```python
from build123d import *

# Parameters (mm, degrees)
F0_W      = 609.6
F0_H      = 609.6
F1_DEPTH  = 482.6
F2_T      = -12.7
F3_DEPTH  = 254
F4_T      = -12.7
F5_W      = 304.8
F5_H      = 609.6
F6_DEPTH  = 469.9
F7_T      = -12.7
F8_DEPTH  = 469.9
F9_DEPTH  = 342.9
F10_W     = 279.4
F10_H     = 457.2
F11_DEPTH = 596.9
F12_W     = 584.2
F12_H     = 330.2
F13_DEPTH = 596.9
F14_W     = 609.6
F14_H     = 1549.4
F15_DEPTH = 12.7


# Not quite as in the source:
# - a shell that OpenCascade refuses in one call is made with other operations: the cavity is built on its own and cut out


with BuildPart() as f1:
    # F0 (on Top) → F1 (new body)
    with BuildSketch(Plane.XY):
        with Locations((3.9980113506, 30.8666436833)):
            Rectangle(F0_W, F0_H)
    extrude(amount=F1_DEPTH)

    # F2
    f2_openings = [f1.faces().sort_by_distance(p)[0] for p in [
        (3.998011, -273.933356, 241.3),
    ]]
    offset(amount=F2_T, openings=f2_openings)

    # F3 (add): a face of the model
    f3_faces = [f1.faces().sort_by_distance(p)[0] for p in [
        (3.9980113506, 30.8666436833, 482.6),
    ]]
    extrude(f3_faces, amount=F3_DEPTH)

    # F4: a shell. OpenCascade refuses it in one call, so the cavity is built on its own and cut out:
    # the body offset inwards by the wall thickness, plus a prism from it out through each open face.
    f4_core = offset(f1.part, amount=F4_T, kind=Kind.INTERSECTION, mode=Mode.PRIVATE)
    f4_exits = [f4_core.faces().sort_by_distance(p)[0] for p in [
        (3.998011, -261.233356, 603.25),
    ]]
    add(f4_core, mode=Mode.SUBTRACT)
    extrude(f4_exits, amount=-F4_T, mode=Mode.SUBTRACT)

    # F5 (on face) → F6 (join)
    with BuildSketch(Plane.XY.offset(736.6)):
        with Locations((-148.4019886494, 30.8666436833)):
            Rectangle(F5_W, F5_H)
    extrude(amount=F6_DEPTH)

    # F7: a shell. OpenCascade refuses it in one call, so the cavity is built on its own and cut out:
    # the body offset inwards by the wall thickness, plus a prism from it out through each open face.
    f7_core = offset(f1.part, amount=F7_T, kind=Kind.INTERSECTION, mode=Mode.PRIVATE)
    f7_exits = [f7_core.faces().sort_by_distance(p)[0] for p in [
        (-148.401989, -261.233356, 965.2),
    ]]
    add(f7_core, mode=Mode.SUBTRACT)
    extrude(f7_exits, amount=-F7_T, mode=Mode.SUBTRACT)

    # F8 (add): a face of the model
    f8_faces = [f1.faces().sort_by_distance(p)[0] for p in [
        (156.3980113506, 30.8666436833, 736.6),
    ]]
    extrude(f8_faces, amount=F8_DEPTH)

    # F9 (add): a face of the model
    f9_faces = [f1.faces().sort_by_distance(p)[0] for p in [
        (3.9980113506, 30.8666436833, 1206.5),
    ]]
    extrude(f9_faces, amount=F9_DEPTH)

    # F10 (on face) → F11 (cut)
    with BuildSketch(Plane.XZ.offset(273.9333563167)):
        with Locations((156.3980113506, 965.2)):
            Rectangle(F10_W, F10_H)
    extrude(amount=-F11_DEPTH, mode=Mode.SUBTRACT)

    # F12 (on face) → F13 (cut)
    with BuildSketch(Plane.XZ.offset(273.9333563167)):
        with Locations((3.9980113506, 1371.6)):
            Rectangle(F12_W, F12_H)
    extrude(amount=-F13_DEPTH, mode=Mode.SUBTRACT)


with BuildPart() as f15:
    # F14 (on face) → F15 (new body)
    with BuildSketch(Plane.XZ.offset(273.9333563167)):
        with Locations((3.9980113506, 774.7)):
            Rectangle(F14_W, F14_H)
    extrude(amount=F15_DEPTH)


solid = f1.part
```
Geometry check sheet. Reference: the model listing, model coordinates, mm. A direction names the side the tool comes from. Coordinates: 2 decimals unless noted, no trailing zeros. Loops run counter-clockwise (first coordinate to the right, second up) from the corner with the lowest first, then second, coordinate; pieces in that order, holes last. Notation, with made-up numbers: (32, 9.25) - (79, 9.25) arc R12 cw to (79, 25.25) - close; hole circle Ø11 at (67, 60.25). An arc over 180 degrees is marked (long way). One line per item, written item: value. Start each with the question number.
(1) Material ranges on line 1 (Z direction, x = 16.5, y = 236); line 2 (Z direction, x = -234.5, y = 271); line 3 (X direction, y = 46, z = 982.5), recorded low to high. Write a range as [from, to].
(2) Cross-section at A-A on y = 174.5. Enter the section's corners in (x, z), plus the area to 3 significant figures.
(3) Depth check by flat-ended pin: P1, Ø12, axis at x = -165.5, z = 1171.5, coming from the -Y side. Enter the tip coordinate at first touch or a pass-through.
(4) Mould release check, pull along Z, two halves, no side actions. Record for faces 1 (the flat face through (0, 35, 0)), 2 (the flat face through (0, 322.967, 238)), 3 (the flat face through (0, 35, 1549.4)), 4 (the flat face through (-150, 29, 736.6)): released by +Z, released by -Z, zero draft, split by the parting line, or undercut.
(5) Tool access check on faces 5 (the flat face through (-300.802, 27, 764)), 6 (the flat face through (0, 20, 1536.7)). Record the directions out of +Z, -Z, +X, -X, +Y, -Y that give a thin tool (end or side, any length) a straight path to the whole face; none if there is none.
(6) Cross-section at B-B on x = 136.5. Enter the section's corners in (y, z), plus the area to 3 significant figures.
(7) Cross-section at C-C on z = 1247.5. Enter the section's corners in (x, y), plus the area to 3 significant figures.
Results below:
1. line 1: z = [0, 12.7], [469.9, 482.6], [723.9, 1206.5], [1536.7, 1549.4]
1. line 2: z = [0, 12.7], [469.9, 482.6], [723.9, 736.6], [1193.8, 1206.5], [1536.7, 1549.4]
1. line 3: x = [-300.8, -288.1], [-8.7, 16.7], [296.1, 308.8]
2. outline: (-300.8, 0) - (308.8, 0) - (308.8, 1549.4) - (-300.8, 1549.4) - close; hole (-288.1, 12.7) - (296.1, 12.7) - (296.1, 469.9) - (-288.1, 469.9) - close; hole (-288.1, 482.6) - (296.1, 482.6) - (296.1, 723.9) - (-288.1, 723.9) - close; hole (-288.1, 736.6) - (-8.7, 736.6) - (-8.7, 1193.8) - (-288.1, 1193.8) - close; hole (-288.1, 1206.5) - (296.1, 1206.5) - (296.1, 1536.7) - (-288.1, 1536.7) - close; hole (16.7, 736.6) - (296.1, 736.6) - (296.1, 1193.8) - (16.7, 1193.8) - close
2. area: 88,100 mm2
3. P1: stops at y = 322.97
4. face 1: released by -Z
4. face 2: undercut
4. face 3: released by +Z
4. face 4: undercut
5. face 5: +Z, -Z, -X, +Y, -Y
5. face 6: -Y
6. outline: (-273.93, 0) - (335.67, 0) - (335.67, 1549.4) - (-273.93, 1549.4) - (-273.93, 1536.7) - (322.97, 1536.7) - (322.97, 1206.5) - (-273.93, 1206.5) - (-273.93, 1193.8) - (322.97, 1193.8) - (322.97, 736.6) - (-273.93, 736.6) - (-273.93, 723.9) - (322.97, 723.9) - (322.97, 482.6) - (-273.93, 482.6) - (-273.93, 469.9) - (322.97, 469.9) - (322.97, 12.7) - (-273.93, 12.7) - close
6. area: 57,600 mm2
7. outline: (-300.8, -273.93) - (-288.1, -273.93) - (-288.1, 322.97) - (296.1, 322.97) - (296.1, -273.93) - (308.8, -273.93) - (308.8, 335.67) - (-300.8, 335.67) - close
7. area: 22,900 mm2
